Input: part model. Units: mm. Frame: model coordinates. Coordinates: 2 decimals unless noted, no trailing zeros. Write each loop counter-clockwise with the first axis right and the second up, starting at its lowest first coordinate (ties: lowest second). Pieces come first, ordered by that corner, then holes. Notation, with made-up numbers: (72.5, 30.25) - (79.5, 30.25) arc R13 ccw to (79.5, 49.25) - close; hole circle Ø2 at (27.25, 57). An arc over 180 degrees is marked (long way). Put each result on its own line as item: value. Start each with the question number.
1. Cut plane C-C, the plane z = -6. Return loops of the section in (x, y) (3 decimals), and give its area (3 significant figures).
2. Pin query (flat end, axial travel): pin 1 (4.5 mm diameter, centred on x = 4.92, z = 0.64, fed in from -Y). Return the tip coordinate at first contact, or that it passes through.
3. Line query: line 1 (X direction, y = -0.4, z = 0.5); line 2 (Z direction, x = -1, y = -0.3) (3 decimals); line 3 (X direction, y = -0.9, z = 0). Output: solid intervals per line, ascending.
4. Cut plane B-B, the plane x = 0. Return loops of the section in (y, z), and give its area (3 significant figures).
5. Cut plane A-A, the plane x = -6.5. Return loops of the section in (y, z), and give its area (3 significant figures).
6. Pull-direction query (X, two-part tool) for faces 1 (the cylindrical face through (6.443, -0.493, 1.269)), 2 (the cylindrical face through (-0.64, -0.49, -11.26)), 3 (the flat face through (1, 0, 0)); classes: released by +X, released by -X, zero draft, split by the parting line, or undercut.
7. Cut plane D-D, the plane z = 2. Return loops of the section in (x, y).
from build123d import *

# Parameters (mm, degrees)
SKETCH1_R           = 12
SKETCH1_R_2         = 1.65
BOSS_EXTRUDE1_DEPTH = 1


with BuildPart() as part:
    # Sketch1 → Boss-Extrude1 (new body)
    with BuildSketch(Plane(origin=(0, 0, 0), x_dir=(1, 0, 0), z_dir=(0, 1, 0))):
        with Locations((0.918840798, -0.637389416)):
            Circle(SKETCH1_R)
        with Locations((-0.138265228, 5.472098091)):
            Circle(SKETCH1_R_2, mode=Mode.SUBTRACT)
        with Locations((-0.138265228, -6.469943597)):
            Circle(SKETCH1_R_2, mode=Mode.SUBTRACT)
        with Locations((-7.081159202, -0.637389416)):
            Circle(SKETCH1_R_2, mode=Mode.SUBTRACT)
        with Locations((4.918840798, -0.637389416)):
            Circle(SKETCH1_R_2, mode=Mode.SUBTRACT)
    extrude(amount=-BOSS_EXTRUDE1_DEPTH)


solid = part.part
Report:
1. outline: (-9.078, -1) - (-1.702, -1) - (-1.702, 0) - (-9.078, 0) - close; (1.425, -1) - (10.916, -1) - (10.916, 0) - (1.425, 0) - close
1. area: 16.9 mm^2
2. pin 1: stops at y = -1
3. line 1: x = -11.08 to -8.73, -5.44 to 3.27, 6.56 to 12.92
3. line 2: z = -11.208 to -6.879, -4.065 to 5.063, 7.877 to 12.483
3. line 3: x = -11.06 to -8.6, -5.56 to 3.4, 6.44 to 12.9
4. outline: (-1, -11.33) - (0, -11.33) - (0, -7.12) - (-1, -7.12) - close; (-1, -3.83) - (0, -3.83) - (0, 4.83) - (-1, 4.83) - close; (-1, 8.11) - (0, 8.11) - (0, 12.6) - (-1, 12.6) - close
4. area: 17.4 mm^2
5. outline: (-1, -8.79) - (0, -8.79) - (0, -0.91) - (-1, -0.91) - close; (-1, 2.18) - (0, 2.18) - (0, 10.07) - (-1, 10.07) - close
5. area: 15.8 mm^2
6. face 1: undercut
6. face 2: split by the parting line
6. face 3: zero draft
7. outline: (-11, -1) - (-8.01, -1) - (-8.01, 0) - (-11, 0) - close; (-6.15, -1) - (3.99, -1) - (3.99, 0) - (-6.15, 0) - close; (5.85, -1) - (12.84, -1) - (12.84, 0) - (5.85, 0) - close
